Geometry: final body of the model. Coordinates: model frame, mm. Round coordinates to 2 decimals unless told otherwise and drop trailing zeros. Loops run counter-clockwise (first coordinate to the right, second up) from the corner with the lowest first, then second, coordinate; pieces in that order, holes last. Notation, with made-up numbers: (85, -23) -> (141, -23) arc R24 cw to (141, 8) -> close; hole circle Ø11 at (47.25, -39.5). An arc over 180 degrees is marked (long way). Answer in a Markdown table with one row per item.
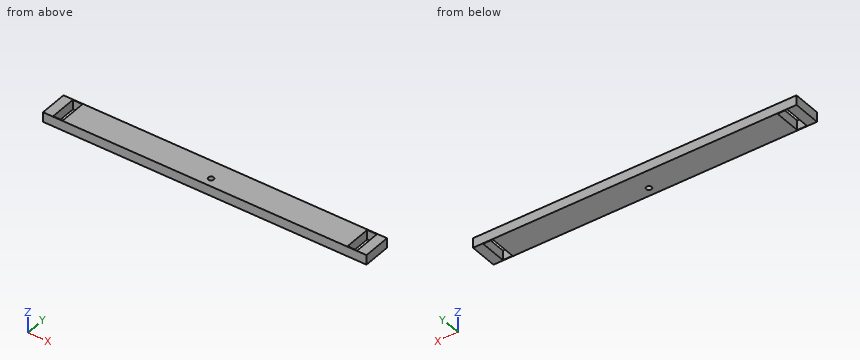
```python
from build123d import *

# Parameters (mm, degrees)
SKETCH1_R           = 5
SKETCH1_W           = 18
SKETCH1_H           = 50
BOSS_EXTRUDE1_DEPTH = 18


with BuildPart() as part:
    # Sketch1 → Boss-Extrude1 (new body)
    with BuildSketch(Plane.XY):
        Polygon((0, 0), (600, 0), (600, -52), (307, -52), (257, -52), (0, -52), align=None)
        with Locations((300, -36)):
            Circle(SKETCH1_R, mode=Mode.SUBTRACT)
        with Locations((573, -26)):
            Rectangle(SKETCH1_W, SKETCH1_H, mode=Mode.SUBTRACT)
        with Locations((27, -26)):
            Rectangle(SKETCH1_W, SKETCH1_H, mode=Mode.SUBTRACT)
    extrude(amount=BOSS_EXTRUDE1_DEPTH)


solid = part.part
```
Item 1: Section query C-C, the plane z = 12. Output: boundary loops of the cut face in (x, y).
Ans:
| item | result |
|---|---|
| outline | (0, -52) -> (600, -52) -> (600, 0) -> (0, 0) -> close; hole (18, -51) -> (36, -51) -> (36, -1) -> (18, -1) -> close; hole circle Ø10 at (300, -36); hole (564, -51) -> (582, -51) -> (582, -1) -> (564, -1) -> close |
Item 2: Ray query, L1, parallel to X at y = -13, z = 7.5; L2, parallel to X at y = -37, z = 12.75; L3, parallel to Y at x = 300, z = 7.5. Return the intervals inside material, ascending.
Ans:
| item | result |
|---|---|
| L1 | 0 to 18, 36 to 564, 582 to 600 |
| L2 | 0 to 18, 36 to 295.1, 304.9 to 564, 582 to 600 |
| L3 | -52 to -41, -31 to 0 |
Item 3: Section query A-A, the plane y = -25.5. Output: boundary loops of the cut face in (x, z).
Ans:
| item | result |
|---|---|
| outline | (0, 0) -> (18, 0) -> (18, 18) -> (0, 18) -> close; (36, 0) -> (564, 0) -> (564, 18) -> (36, 18) -> close; (582, 0) -> (600, 0) -> (600, 18) -> (582, 18) -> close |
Item 4: Section query B-B, the plane x = 300. Output: boundary loops of the cut face in (y, z), and give its area (3 significant figures).
Ans:
| item | result |
|---|---|
| outline | (-52, 0) -> (-41, 0) -> (-41, 18) -> (-52, 18) -> close; (-31, 0) -> (0, 0) -> (0, 18) -> (-31, 18) -> close |
| area | 756 mm2 |
